Model file for the job. Use its own axes, mm. Round coordinates to 2 decimals unless told otherwise and drop trailing zeros. Order: outer loops, then holes, each group sorted by start corner. A loop starts at its lowest first (then second) coordinate and runs counter-clockwise, first axis right, second up. Notation, with made-up numbers: (30.5, -29.5) -> (76.5, -29.5) arc R21 cw to (76.5, -4.5) -> close; hole circle Ø10 at (35, 54.25). An arc over 180 degrees is marked (long way). Answer as CSV lines item,"result".
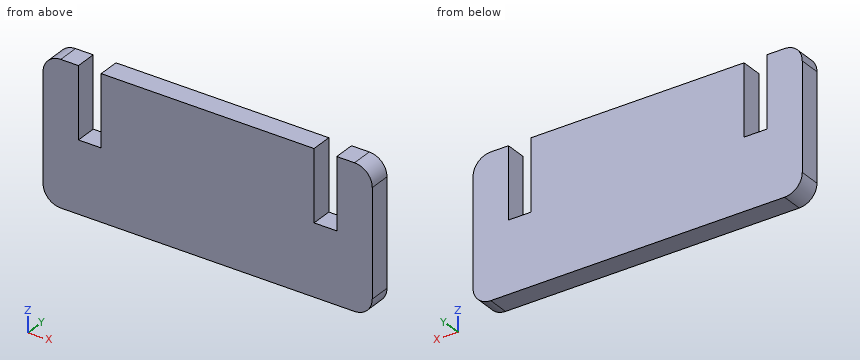
```python
from build123d import *

# Parameters (mm, degrees)
EXTRUDE_1_DEPTH = 3


with BuildPart() as part:
    # 草图1 → 凸台-拉伸1 (new body)
    with BuildSketch(Plane(origin=(0, 0, 0), x_dir=(1, 0, 0), z_dir=(0, 1, 0))):
        with BuildLine():
            Line((15, 10), (20.7, 10))
            ThreePointArc((20.7, 10), (22.467766953, 9.267766953), (23.2, 7.5))
            Line((23.2, 7.5), (23.2, -7.5))
            ThreePointArc((23.2, -7.5), (22.467766953, -9.267766953), (20.7, -10))
            Line((20.7, -10), (18.2, -10))
            Line((18.2, -10), (18.2, 0))
            Line((18.2, 0), (15, 0))
            Line((15, 0), (15, -10))
            Line((15, -10), (-15, -10))
            Line((-15, -10), (-15, 0))
            Line((-15, 0), (-18.2, 0))
            Line((-18.2, 0), (-18.2, -10))
            Line((-18.2, -10), (-20.7, -10))
            ThreePointArc((-20.7, -10), (-22.467766953, -9.267766953), (-23.2, -7.5))
            Line((-23.2, -7.5), (-23.2, 7.5))
            ThreePointArc((-23.2, 7.5), (-22.467766953, 9.267766953), (-20.7, 10))
            Line((-20.7, 10), (-15, 10))
            Line((-15, 10), (15, 10))
        make_face()
    extrude(amount=EXTRUDE_1_DEPTH)


solid = part.part
```
Q1. Wall check: L1, parallel to X at y = 0.3, z = 7; L2, parallel to X at y = 0.3, z = 9; L3, parallel to Z at x = 18, y = 2.15. Give the ranges that are in metal, low to high. Write a range as [from, to].
Checks:
L1,"[-23.2, -18.2], [-15, 15], [18.2, 23.2]"
L2,"[-22.7, -18.2], [-15, 15], [18.2, 22.7]"
L3,"[-10, 0]"
Q2. Flat gauge pin, fed straight in: pin 1 (0.9 mm diameter, centred on x = -16.5, y = 2, fed in from +Z). Where does the tip first touch, or does it go through?
Checks:
pin 1,"z = 0"
Q3. Saw through at C-C (x = 17.5). Write the cut outline in (y, z).
Checks:
outline,"(0, -10) -> (3, -10) -> (3, 0) -> (0, 0) -> close"
Q4. Saw through at A-A (z = 4.5). Write the cut outline in (x, y).
Checks:
outline,"(-23.2, 0) -> (-18.2, 0) -> (-18.2, 3) -> (-23.2, 3) -> close; (-15, 0) -> (15, 0) -> (15, 3) -> (-15, 3) -> close; (18.2, 0) -> (23.2, 0) -> (23.2, 3) -> (18.2, 3) -> close"
Q5. Saw through at B-B (y = 1.6). Write the cut outline in (x, z), plus the area to 3 significant figures.
Checks:
outline,"(-23.2, -7.5) arc R2.5 ccw to (-20.7, -10) -> (20.7, -10) arc R2.5 ccw to (23.2, -7.5) -> (23.2, 7.5) arc R2.5 ccw to (20.7, 10) -> (18.2, 10) -> (18.2, 0) -> (15, 0) -> (15, 10) -> (-15, 10) -> (-15, 0) -> (-18.2, 0) -> (-18.2, 10) -> (-20.7, 10) arc R2.5 ccw to (-23.2, 7.5) -> close"
area,"859 mm²"
